Design review of the part built by this model. Coordinates are the model's own, in mm. A direction names the side the tool comes from. Give positions to 0.01 mm unless a question says otherwise; leave off trailing zeros. Loops run counter-clockwise (first coordinate to the right, second up) from the corner with the lowest first, then second, coordinate; pieces in that order, holes last. Notation, with made-up numbers: (3, 81) - (57, 81) arc R23 cw to (57, 94) - close; hole circle Ø8 at (34, 8). An arc over 180 degrees is marked (long way). Write each question's results on one line, items separated by ' | '.
from build123d import *

# Parameters (mm, degrees)
SKETCH1_W           = 3.175
SKETCH1_H           = 15.875
BOSS_EXTRUDE1_DEPTH = 77
SKETCH2_W           = 10
SKETCH2_H           = 3.175
BOSS_EXTRUDE2_DEPTH = 3.175


with BuildPart() as part:
    # Sketch1 → Boss-Extrude1 (new body)
    with BuildSketch(Plane(origin=(0, 0, 0), x_dir=(0, 0, -1), z_dir=(1, 0, 0))):
        with Locations((-0.564444444, 7.9375)):
            Rectangle(SKETCH1_W, SKETCH1_H)
    extrude(amount=BOSS_EXTRUDE1_DEPTH)

    # Sketch2 → Boss-Extrude2 (add)
    with BuildSketch(Plane(origin=(0, 0, -1.023055556), x_dir=(-1, 0, 0), z_dir=(0, 0, -1))):
        with Locations((-52, -1.5875)):
            Rectangle(SKETCH2_W, SKETCH2_H)
        with Locations((-72, -1.5875)):
            Rectangle(SKETCH2_W, SKETCH2_H)
        with Locations((-32, -1.5875)):
            Rectangle(SKETCH2_W, SKETCH2_H)
        with Locations((-12, -1.5875)):
            Rectangle(SKETCH2_W, SKETCH2_H)
    extrude(amount=-BOSS_EXTRUDE2_DEPTH)


solid = part.part
(1) Take a section at A-A on y = -1. Give the boundary of the cut face in (x, z), plus the area to 3 significant figures.
Answers below:
outline: (7, -1.02) - (17, -1.02) - (17, 2.15) - (7, 2.15) - close; (27, -1.02) - (37, -1.02) - (37, 2.15) - (27, 2.15) - close; (47, -1.02) - (57, -1.02) - (57, 2.15) - (47, 2.15) - close; (67, -1.02) - (77, -1.02) - (77, 2.15) - (67, 2.15) - close | area: 127 mm2
(2) Take a section at C-C on x = 5. Give the boundary of the cut face in (y, z) (3 decimals).
Answers below:
outline: (0, -1.023) - (15.875, -1.023) - (15.875, 2.152) - (0, 2.152) - close
(3) Insertion check: P1, Ø1.6, axis at y = -1.5, z = 0.5, coming from the -X side; P2, Ø1, axis at x = 3, z = 1.5, coming from the -Y side. Each pin has a flat end and moves straight along its axis. Give the tip position at first contact, or say it passes through.
Answers below:
P1: x = 7 | P2: y = 0
(4) Take a section at B-B on z = 1. Give the boundary of the cut face in (x, y) (3 decimals), plus the area to 3 significant figures.
Answers below:
outline: (0, 0) - (7, 0) - (7, -3.175) - (17, -3.175) - (17, 0) - (27, 0) - (27, -3.175) - (37, -3.175) - (37, 0) - (47, 0) - (47, -3.175) - (57, -3.175) - (57, 0) - (67, 0) - (67, -3.175) - (77, -3.175) - (77, 15.875) - (0, 15.875) - close | area: 1,350 mm2
(5) Tool access review of faces 1 (the flat face through (12, -3.175, 1)), 2 (the flat face through (67, -2, 1)), 3 (the flat face through (7, -2, 1)): name each direction out of +Z, -Z, +X, -X, +Y, -Y from which nothing blocks a thin tool from reaching the whole face with its end or side.
Answers below:
face 1: +Z, -Z, +X, -X, -Y | face 2: +Z, -Z, -Y | face 3: +Z, -Z, -X, -Y
(6) Wall thickness on line 1 along X through (y, z) = (-1, -0.3); line 2 along Y through (x, z) = (20.5, -0.65) (3 decimals): over which ranges is each line inside the solid? List them lowest first. Write a range as from..to.
Answers below:
line 1: 7..17, 27..37, 47..57, 67..77 | line 2: 0..15.875
(7) Draft analysis for pull direction X (two halves, no side actions). For faces 4 (the flat face through (38, 15.875, 1)), 5 (the flat face through (77, 6, 1)), 6 (the flat face through (17, -2, 1)), state which applies: pulls with the +X half, pulls with the -X half, needs draft (parallel to the pull), parting line crosses it, or undercut.
Answers below:
face 4: needs draft | face 5: pulls with the +X half | face 6: undercut
